```python
from build123d import *

# Parameters (mm, degrees)
BOSS_EXTRUDE1_DEPTH             = 5
F_3_0MM_DOWEL_HOLE1_D           = 2.8
F_3_0MM_DOWEL_HOLE1_DEPTH       = 10
F_3_0MM_DOWEL_HOLE1_CSINK_D     = 4
F_3_0MM_DOWEL_HOLE1_CSINK_ANGLE = 90
F_3_0MM_DOWEL_HOLE1_TIP         = 0.841204867
F_2_5MM_DOWEL_HOLE1_D           = 2.3
F_2_5MM_DOWEL_HOLE1_DEPTH       = 10
F_2_5MM_DOWEL_HOLE1_TIP         = 0.690989712
CUT_EXTRUDE1_REACH              = 68.046
SKETCH6_W                       = 3
SKETCH6_H                       = 3
FILLET2_R                       = 2
CHAMFER1_SIZE                   = 1


with BuildPart() as part:
    # Sketch1 → Boss-Extrude1 (new body)
    with BuildSketch(Plane.XY):
        Polygon((0, 0), (-25, 0), (-25, 3), (-33, 3), (-32, -56.991666088), (-26, -56.991666088), (-26, -4), (0, -4), align=None)
    extrude(amount=BOSS_EXTRUDE1_DEPTH)

    # Ø3.0mm Dowel Hole1
    with Locations(Plane(origin=(0, -56.991666088, 0), x_dir=(-1, 0, 0), z_dir=(0, -1, 0))):
        with Locations((29, -2.5)):
            CounterSinkHole(F_3_0MM_DOWEL_HOLE1_D / 2, F_3_0MM_DOWEL_HOLE1_CSINK_D / 2, depth=F_3_0MM_DOWEL_HOLE1_DEPTH, counter_sink_angle=F_3_0MM_DOWEL_HOLE1_CSINK_ANGLE)
            with Locations((0, 0, -(F_3_0MM_DOWEL_HOLE1_DEPTH + F_3_0MM_DOWEL_HOLE1_TIP / 2))):  # 118° drill point
                Cone(0, F_3_0MM_DOWEL_HOLE1_D / 2, F_3_0MM_DOWEL_HOLE1_TIP, mode=Mode.SUBTRACT)

    # Mirror1: part across plane


with BuildPart() as part_1:
    add(part.part)
    add(part.part.mirror(Plane(origin=(0, -4, 5), x_dir=(0, 0, 1), z_dir=(-1, 0, 0))))

    # Ø2.5mm Dowel Hole1
    with Locations(Plane(origin=(0, 3, 0), x_dir=(1, 0, 0), z_dir=(0, 1, 0))):
        with Locations((-30.5, -2.5), (27.5, -2.5)):
            Hole(F_2_5MM_DOWEL_HOLE1_D / 2, depth=F_2_5MM_DOWEL_HOLE1_DEPTH)
            with Locations((0, 0, -(F_2_5MM_DOWEL_HOLE1_DEPTH + F_2_5MM_DOWEL_HOLE1_TIP / 2))):  # 118° drill point
                Cone(0, F_2_5MM_DOWEL_HOLE1_D / 2, F_2_5MM_DOWEL_HOLE1_TIP, mode=Mode.SUBTRACT)

    # Sketch6 → Cut-Extrude1 (cut, up to next)
    with BuildSketch(Plane.XY.offset(5), mode=Mode.PRIVATE) as cut_extrude1_sk1:
        with Locations((-26.5, 1.5)):
            Rectangle(SKETCH6_W, SKETCH6_H)
    cut_extrude1_tool1 = extrude(cut_extrude1_sk1.sketch, amount=-CUT_EXTRUDE1_REACH, mode=Mode.PRIVATE) & part_1.part
    # Sketch6 → Cut-Extrude1 (cut, up to next)
    with BuildSketch(Plane.XY.offset(5), mode=Mode.PRIVATE) as cut_extrude1_sk2:
        with Locations((31.5, 1.5)):
            Rectangle(SKETCH6_W, SKETCH6_H)
    cut_extrude1_tool2 = extrude(cut_extrude1_sk2.sketch, amount=-CUT_EXTRUDE1_REACH, mode=Mode.PRIVATE) & part_1.part
    add(cut_extrude1_tool1.solids().sort_by_distance((-26.5, 1.5, 5))[0], mode=Mode.SUBTRACT)
    add(cut_extrude1_tool2.solids().sort_by_distance((31.5, 1.5, 5))[0], mode=Mode.SUBTRACT)

    # Fillet2
    fillet2_edges = [part_1.edges().sort_by_distance(p)[0] for p in [
        (-26, -4, 2.5),
        (25, 0, 2.5),
        (26, -4, 2.5),
        (-28, 0, 2.5),
        (30, 0, 2.5),
    ]]
    fillet(fillet2_edges, radius=FILLET2_R)

    # Chamfer1
    # the kernel refuses this chamfer: 1 mm, written as the material it takes off along each edge
    with BuildSketch(Plane(origin=(32, 2, 5), x_dir=(0, -1, 0), z_dir=(1, 0, 0))) as chamfer1_piece_1:
        Polygon((2 + CHAMFER1_SIZE, 0), (2, CHAMFER1_SIZE), (2, 0), align=None)
    revolve(axis=Axis((32, 2, 5), (0, 0, -1)), revolution_arc=90, mode=Mode.SUBTRACT)
    with BuildSketch(Plane(origin=(32, 2, 0), x_dir=(0, -1, 0), z_dir=(1, 0, 0))) as chamfer1_piece_2:
        Polygon((2 + CHAMFER1_SIZE, 0), (2, -CHAMFER1_SIZE), (2, 0), align=None)
    revolve(axis=Axis((32, 2, 0), (0, 0, -1)), revolution_arc=90, mode=Mode.SUBTRACT)
    with BuildSketch(Plane(origin=(-26, 2, 5), x_dir=(0, -1, 0), z_dir=(1, 0, 0))) as chamfer1_piece_3:
        Polygon((2, CHAMFER1_SIZE), (2 + CHAMFER1_SIZE, 0), (2, 0), align=None)
    revolve(axis=Axis((-26, 2, 5), (0, 0, -1)), revolution_arc=90, mode=Mode.SUBTRACT)
    with BuildSketch(Plane(origin=(-26, 2, 0), x_dir=(0, -1, 0), z_dir=(1, 0, 0))) as chamfer1_piece_4:
        Polygon((2 + CHAMFER1_SIZE, 0), (2, -CHAMFER1_SIZE), (2, 0), align=None)
    revolve(axis=Axis((-26, 2, 0), (0, 0, -1)), revolution_arc=90, mode=Mode.SUBTRACT)
    with BuildSketch(Plane(origin=(24, -6, 0), x_dir=(0, 1, 0), z_dir=(-1, 0, 0))) as chamfer1_piece_5:
        Polygon((2 + CHAMFER1_SIZE, 0), (2, -CHAMFER1_SIZE), (2, 0), align=None)
    revolve(axis=Axis((24, -6, 0), (0, 0, -1)), revolution_arc=90, mode=Mode.SUBTRACT)
    with BuildSketch(Plane(origin=(24, -6, 5), x_dir=(0, 1, 0), z_dir=(-1, 0, 0))) as chamfer1_piece_6:
        Polygon((2 + CHAMFER1_SIZE, 0), (2, CHAMFER1_SIZE), (2, 0), align=None)
    revolve(axis=Axis((24, -6, 5), (0, 0, -1)), revolution_arc=90, mode=Mode.SUBTRACT)
    with BuildSketch(Plane(origin=(-24, -6, 0), x_dir=(-1, 0, 0), z_dir=(0, -1, 0))) as chamfer1_piece_7:
        Polygon((2 + CHAMFER1_SIZE, 0), (2, -CHAMFER1_SIZE), (2, 0), align=None)
    revolve(axis=Axis((-24, -6, 0), (0, 0, -1)), revolution_arc=90, mode=Mode.SUBTRACT)
    with BuildSketch(Plane(origin=(-24, -6, 5), x_dir=(-1, 0, 0), z_dir=(0, -1, 0))) as chamfer1_piece_8:
        Polygon((2 + CHAMFER1_SIZE, 0), (2, CHAMFER1_SIZE), (2, 0), align=None)
    revolve(axis=Axis((-24, -6, 5), (0, 0, -1)), revolution_arc=90, mode=Mode.SUBTRACT)
    with BuildSketch(Plane(origin=(23, 2, 0), x_dir=(0, -1, 0), z_dir=(-1, 0, 0))) as chamfer1_piece_9:
        Polygon((2 + CHAMFER1_SIZE, 0), (2, CHAMFER1_SIZE), (2, 0), align=None)
    revolve(axis=Axis((23, 2, 0), (0, 0, 1)), revolution_arc=90, mode=Mode.SUBTRACT)
    with BuildSketch(Plane(origin=(23, 2, 5), x_dir=(0, -1, 0), z_dir=(-1, 0, 0))) as chamfer1_piece_10:
        Polygon((2, -CHAMFER1_SIZE), (2 + CHAMFER1_SIZE, 0), (2, 0), align=None)
    revolve(axis=Axis((23, 2, 5), (0, 0, 1)), revolution_arc=90, mode=Mode.SUBTRACT)
    with BuildSketch(Plane(origin=(-33.042861383, 5.571325785, 5), x_dir=(0.9994830708911936, 0.016660365281854946, 0.027495876610586452), z_dir=(0.01666666666666667, -0.9998611014647096, 0))) as chamfer1_piece_11:
        Polygon((CHAMFER1_SIZE * 0.999621916911, -CHAMFER1_SIZE * 0.0274958766106), (-CHAMFER1_SIZE * 0.0274958766106, -CHAMFER1_SIZE * 0.999621916911), (0, 0), align=None)
    extrude(amount=65.143365976, mode=Mode.SUBTRACT)
    with BuildSketch(Plane(origin=(-26, -59.563349076, 5), x_dir=(-0.9996219169112968, 0, 0.02749587661058651), z_dir=(0, 1, 0)), Plane(origin=(26, -59.563349076, 0), x_dir=(0.9996219169112968, 0, -0.02749587661058634), z_dir=(0, 1, 0))) as chamfer1_piece_12:
        Polygon((CHAMFER1_SIZE * 0.999621916911, -CHAMFER1_SIZE * 0.0274958766106), (-CHAMFER1_SIZE * 0.0274958766106, -CHAMFER1_SIZE * 0.999621916911), (0, 0), align=None)
    extrude(amount=53.563349076, mode=Mode.SUBTRACT)
    with BuildSketch(Plane(origin=(26, -59.563349076, 5), x_dir=(0.9996219169112968, 0, 0.02749587661058651), z_dir=(0, 1, 0)), Plane(origin=(-26, -59.563349076, 0), x_dir=(-0.9996219169112968, 0, -0.02749587661058639), z_dir=(0, 1, 0))) as chamfer1_piece_13:
        Polygon((CHAMFER1_SIZE * 0.999621916911, CHAMFER1_SIZE * 0.0274958766106), (-CHAMFER1_SIZE * 0.0274958766106, CHAMFER1_SIZE * 0.999621916911), (0, 0), align=None)
    extrude(amount=53.563349076, mode=Mode.SUBTRACT)
    with BuildSketch(Plane(origin=(32.992854437, 2.571325785, 0), x_dir=(-0.9994830708911936, 0.016660365281854946, -0.02749587661058633), z_dir=(-0.01666666666666667, -0.9998611014647096, 0))) as chamfer1_piece_14:
        Polygon((CHAMFER1_SIZE * 0.999621916911, -CHAMFER1_SIZE * 0.0274958766106), (-CHAMFER1_SIZE * 0.0274958766106, -CHAMFER1_SIZE * 0.999621916911), (0, 0), align=None)
    extrude(amount=62.142949222, mode=Mode.SUBTRACT)
    with BuildSketch(Plane(origin=(32.992854437, 2.571325785, 5), x_dir=(-0.9994830708911936, 0.016660365281854946, 0.027495876610586452), z_dir=(-0.01666666666666667, -0.9998611014647096, 0))) as chamfer1_piece_15:
        Polygon((CHAMFER1_SIZE * 0.999621916911, CHAMFER1_SIZE * 0.0274958766106), (-CHAMFER1_SIZE * 0.0274958766106, CHAMFER1_SIZE * 0.999621916911), (0, 0), align=None)
    extrude(amount=62.142949222, mode=Mode.SUBTRACT)
    with BuildSketch(Plane(origin=(-28, 5.571682988, 5), x_dir=(-0.9996219169112968, 0, 0.02749587661058651), z_dir=(0, -1, 0)), Plane(origin=(30, 5.571682988, 5), x_dir=(-0.9996219169112968, 0, 0.02749587661058651), z_dir=(0, -1, 0)), Plane(origin=(30, 2, 0), x_dir=(-0.9996219169112968, 0, -0.02749587661058634), z_dir=(0, 1, 0)), Plane(origin=(-28, 2, 0), x_dir=(-0.9996219169112968, 0, -0.02749587661058639), z_dir=(0, 1, 0)), Plane(origin=(25, 2, 5), x_dir=(0.9996219169112968, 0, 0.027495876610586605), z_dir=(0, 1, 0))) as chamfer1_piece_16:
        Polygon((CHAMFER1_SIZE * 0.999621916911, CHAMFER1_SIZE * 0.0274958766106), (-CHAMFER1_SIZE * 0.0274958766106, CHAMFER1_SIZE * 0.999621916911), (0, 0), align=None)
    extrude(amount=3.571682988, mode=Mode.SUBTRACT)
    with BuildSketch(Plane(origin=(-33.042861383, 5.571325785, 0), x_dir=(0.9994830708911936, 0.016660365281854946, -0.02749587661058633), z_dir=(0.01666666666666667, -0.9998611014647096, 0))) as chamfer1_piece_17:
        Polygon((CHAMFER1_SIZE * 0.999621916911, CHAMFER1_SIZE * 0.0274958766106), (-CHAMFER1_SIZE * 0.0274958766106, CHAMFER1_SIZE * 0.999621916911), (0, 0), align=None)
    extrude(amount=65.143365976, mode=Mode.SUBTRACT)
    with BuildSketch(Plane(origin=(23, 0, 0), x_dir=(0, 0.02749587661059217, 0.9996219169112965), z_dir=(-1, 0, 0)), Plane(origin=(-26, 0, 5), x_dir=(0, 0.027495876610583284, -0.9996219169112968), z_dir=(1, 0, 0))) as chamfer1_piece_18:
        Polygon((CHAMFER1_SIZE * 0.999621916911, -CHAMFER1_SIZE * 0.0274958766106), (-CHAMFER1_SIZE * 0.0274958766106, -CHAMFER1_SIZE * 0.999621916911), (0, 0), align=None)
    extrude(amount=49, mode=Mode.SUBTRACT)
    with BuildSketch(Plane(origin=(24, -4, 0), x_dir=(0, 0.9996219169112968, -0.027495876610586365), z_dir=(-1, 0, 0)), Plane(origin=(-24, -4, 5), x_dir=(0, 0.9996219169112968, 0.027495876610586487), z_dir=(1, 0, 0))) as chamfer1_piece_19:
        Polygon((CHAMFER1_SIZE * 0.999621916911, -CHAMFER1_SIZE * 0.0274958766106), (-CHAMFER1_SIZE * 0.0274958766106, -CHAMFER1_SIZE * 0.999621916911), (0, 0), align=None)
    extrude(amount=48, mode=Mode.SUBTRACT)
    with BuildSketch(Plane(origin=(25, 2, 0), x_dir=(0.9996219169112968, 0, -0.02749587661058654), z_dir=(0, 1, 0))) as chamfer1_piece_20:
        Polygon((CHAMFER1_SIZE * 0.999621916911, -CHAMFER1_SIZE * 0.0274958766106), (-CHAMFER1_SIZE * 0.0274958766106, -CHAMFER1_SIZE * 0.999621916911), (0, 0), align=None)
    extrude(amount=3.571682988, mode=Mode.SUBTRACT)
    with BuildSketch(Plane(origin=(35.521676042, 0, 0), x_dir=(0, -0.9996219169112968, -0.027495876610586365), z_dir=(-1, 0, 0)), Plane(origin=(32, 0, 5), x_dir=(0, -0.9996219169112968, 0.027495876610586497), z_dir=(1, 0, 0))) as chamfer1_piece_21:
        Polygon((CHAMFER1_SIZE * 0.999621916911, CHAMFER1_SIZE * 0.0274958766106), (-CHAMFER1_SIZE * 0.0274958766106, CHAMFER1_SIZE * 0.999621916911), (0, 0), align=None)
    extrude(amount=3.521676042, mode=Mode.SUBTRACT)


solid = part_1.part
```
Geometry check sheet. Reference: the model listing, model coordinates, mm. A direction names the side the tool comes from. Give positions to 0.01 mm unless a question says otherwise; leave off trailing zeros. Loops run counter-clockwise (first coordinate to the right, second up) from the corner with the lowest first, then second, coordinate; pieces in that order, holes last. Notation, with made-up numbers: (73.25, 57) - (106.25, 57) arc R32 cw to (106.25, 84) - close; hole circle Ø11 at (83, 23.5). An arc over 180 degrees is marked (long way). Use CSV: the item, a comma, the result in double quotes. Start each with the question number.
Q1. Access from +Z, -Z, +X, -X, +Y, -Y to the whole of each face (thin tool, end or side, straight path). Record for faces 1 (the face through (-27.68, 0.29, 4.4)), 2 (the face through (29.232, -46.297, 2.427)), 3 (the face through (25.666, -4.297, 0.618)), 4 (the face through (-25.43, -4.6, 2.52)).
Q2. Go/stop test with flat-tipped pins: pin 1 Ø3 at (x, z) = (-29, 2.5) entering from -Y; pin 2 Ø2.5 at (x, z) = (10.5, 2) entering from -Y; pin 3 Ø1.5 at (y, z) = (-39, 2.5) entering from +X. Record where each tip stops, or that it passes through.
Q3. Section check B-B, the plane x = -9. Record the cut outline in (y, z), and give its area (3 significant figures).
Q4. Section check A-A, the plane y = -50.5. Record the cut outline in (x, z).
Q5. Release check for a two-part mould opening along Z. For faces 5 (the face through (30.4, -51.63, 2.44)), 6 (the face through (27.3, -7.57, 2.49)), 7 (the face through (30.334, 0.297, 0.618)), 8 (the face through (26, -32, 2)) record: +Z half, -Z half, draft (parallel to the pull), parting line (faces both ways), or undercut.
Q6. Section check C-C, the plane y = -44. Record the cut outline in (x, z).
Q7. Scan lines: probe 1 along Z at (x, y) = (29, -52); probe 2 along Z at (x, y) = (-30.5, -3.5); probe 3 along Y at (x, z) = (23, 1.1). Record each from-to range of solid material in increasing order. Write a range as from..to.
Findings below:
1,face 1,"+Z, +Y"
1,face 2,"-Y"
1,face 3,"-Z, -Y"
1,face 4,"+Z, -Z, -Y"
2,pin 1,"stops at y = -56.49"
2,pin 2,"stops at y = -4"
2,pin 3,"stops at x = 32.31"
3,outline,"(-4, 1) - (-3, 0) - (-1, 0) - (0, 1) - (0, 4) - (-1, 5) - (-3, 5) - (-4, 4) - close"
3,area,"18.0 mm^2"
4,outline,"(-32.11, 1) - (-31.11, 0) - (-27, 0) - (-26, 1) - (-26, 4) - (-27, 5) - (-31.11, 5) - (-32.11, 4) - close; (26, 1) - (27, 0) - (31.11, 0) - (32.11, 1) - (32.11, 4) - (31.11, 5) - (27, 5) - (26, 4) - close; hole circle Ø2.8 at (-29, 2.5); hole circle Ø2.8 at (29, 2.5)"
5,face 5,"undercut"
5,face 6,"undercut"
5,face 7,"-Z half"
5,face 8,"draft"
6,outline,"(-32.22, 1) - (-31.22, 0) - (-27, 0) - (-26, 1) - (-26, 4) - (-27, 5) - (-31.22, 5) - (-32.22, 4) - close; (26, 1) - (27, 0) - (31.22, 0) - (32.22, 1) - (32.22, 4) - (31.22, 5) - (27, 5) - (26, 4) - close"
7,probe 1,"z = 0..1.1, 3.9..5"
7,probe 2,"z = 0..1.35, 3.65..5"
7,probe 3,"y = -4..0"
